Source: CAD feature listing. Evaluate the final solid. Frame: model axes, mm. Face numbers are marked on the shaded views. A direction names the side the tool comes from. Coordinates: 2 decimals unless noted, no trailing zeros. Loops run counter-clockwise (first coordinate to the right, second up) from the corner with the lowest first, then second, coordinate; pieces in that order, holes last. Notation, with made-up numbers: (73.25, 16) -> (107.25, 16) arc R23 cw to (107.25, 35) -> close; hole circle Ø4 at (23.25, 0.25). An arc over 180 degrees is marked (long way). One line per question, with ' | ' between items. Start each with the question number.
```python
from build123d import *

# Parameters (mm, degrees)
F0_W      = 1600
F0_H      = 1600
F2_DEPTH  = 150
F1_W      = 1250
F1_H      = 1250
F1_W_2    = 1150
F1_H_2    = 1150
F3_DEPTH  = 1250
F4_W      = 1250
F4_H      = 1250
F4_W_2    = 450
F4_H_2    = 450
F5_DEPTH  = 50
F6_W      = 550
F6_H      = 550
F6_W_2    = 450
F6_H_2    = 450
F7_DEPTH  = 100
F8_R      = 27.85
F9_DEPTH  = 100
F10_R     = 27.85
F11_DEPTH = 200


with BuildPart() as f2:
    # F0 (on Top) → F2 (new body)
    with BuildSketch(Plane.XY):
        Rectangle(F0_W, F0_H)
    extrude(amount=-F2_DEPTH)

    # F1 (on Top) → F3 (join)
    with BuildSketch(Plane.XY):
        Rectangle(F1_W, F1_H)
        Rectangle(F1_W_2, F1_H_2, mode=Mode.SUBTRACT)
    extrude(amount=F3_DEPTH)

    # F4 (on face) → F5 (join)
    with BuildSketch(Plane.XY.offset(1250)):
        Rectangle(F4_W, F4_H)
        with Locations((-350, 0)):
            Rectangle(F4_W_2, F4_H_2, mode=Mode.SUBTRACT)
    extrude(amount=F5_DEPTH)

    # F6 (on face) → F7 (join)
    with BuildSketch(Plane.XY.offset(1300)):
        with Locations((-350, 0)):
            Rectangle(F6_W, F6_H)
        with Locations((-350, 0)):
            Rectangle(F6_W_2, F6_H_2, mode=Mode.SUBTRACT)
    extrude(amount=F7_DEPTH)

    # F8 (on face) → F9 (cut)
    with BuildSketch(Plane.YZ.offset(625)):
        with Locations((0, 800)):
            Circle(F8_R)
    extrude(amount=-F9_DEPTH, mode=Mode.SUBTRACT)

    # F10 (on face) → F11 (cut)
    with BuildSketch(Plane(origin=(0, 0, -150), x_dir=(1, 0, 0), z_dir=(0, 0, -1))):
        with Locations((-125, -150)):
            Circle(F10_R)
        with Locations((-225, 150)):
            Circle(F10_R)
    extrude(amount=-F11_DEPTH, mode=Mode.SUBTRACT)


solid = f2.part
```
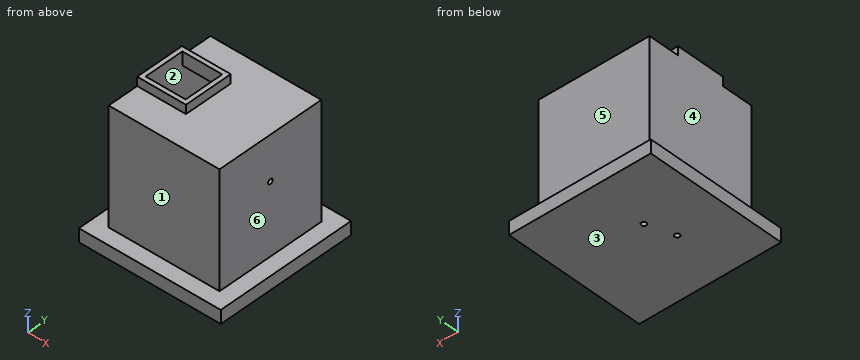
(1) Cut plane B-B, the plane x = 419. Return the cut outline in (y, z).
(2) Cut plane A-A, the plane y = 0. Return the cut outline in (x, z), and give its area (3 significant figures).
(3) Cut plane D-D, the plane z = 800. Return the cut outline in (x, y).
(4) Draft query along Z for the marked faces 1, 2 and 3. Return one class per face: pulls with the +Z half, pulls with the -Z half, needs draft (parallel to the pull), parting line crosses it, or undercut.
(5) Contact query for flat-ended pins moving along their axis: pin 1 Ø2 at (x, z) = (-369, 589.5) entering from -Y; pin 2 Ø1.5 at (x, y) = (5.5, -271) entering from +Z; pin 3 Ø8 at (x, z) = (-342, 141) entering from +Y. Output: stop coordinate, or through.
(6) Access query for the marked faces 4, 5 and 6. Directions: +Z, -Z, +X, -X, +Y, -Y. A direction counts if a zero-diameter tool reaches every point of the face in a straight line with its end or side. Return the directions, or none.
(7) Ray query, L1, parallel to X at y = 391, z = 361; L2, parallel to Z at x = 598, y = 0. Return the intervals inside material, ascending.
Here are the results:
1) outline: (-800, -150) -> (800, -150) -> (800, 0) -> (625, 0) -> (625, 1300) -> (-625, 1300) -> (-625, 0) -> (-800, 0) -> close; hole (-575, 0) -> (575, 0) -> (575, 1250) -> (-575, 1250) -> close
2) outline: (-800, -150) -> (800, -150) -> (800, 0) -> (625, 0) -> (625, 772.15) -> (575, 772.15) -> (575, 0) -> (-575, 0) -> (-575, 1400) -> (-625, 1400) -> (-625, 0) -> (-800, 0) -> close; (-125, 1250) -> (575, 1250) -> (575, 827.85) -> (625, 827.85) -> (625, 1300) -> (-75, 1300) -> (-75, 1400) -> (-125, 1400) -> close | area: 412,000 mm2
3) outline: (-625, -625) -> (625, -625) -> (625, -27.85) -> (575, -27.85) -> (575, -575) -> (-575, -575) -> (-575, 575) -> (575, 575) -> (575, 27.85) -> (625, 27.85) -> (625, 625) -> (-625, 625) -> close
4) face 1: needs draft | face 2: undercut | face 3: pulls with the -Z half
5) pin 1: stops at y = -625 | pin 2: stops at z = 1300 | pin 3: stops at y = 625
6) face 4: +Z, -X, +Y, -Y | face 5: +Z, +X, -X, +Y | face 6: +Z, +X, +Y, -Y
7) L1: x = -625 to -575, 575 to 625 | L2: z = -150 to 772.15, 827.85 to 1300
